Check sheet for the modelled part. Datum: model origin and axes. Units: mm. A direction names the side the tool comes from. Coordinates: 2 decimals unless noted, no trailing zeros. Loops run counter-clockwise (first coordinate to the right, second up) from the corner with the lowest first, then second, coordinate; pieces in that order, holes last. Notation, with made-up numbers: M 30,74 L 48,74 A17 cw 48,100 Z; hole C -3,-3.5 d1. An arc over 180 degrees is marked long. Use CSV: the item, a comma, the result in double quotes. Start each with the question number.
(1) Scan lines: line 1 (X direction, y = 2, z = 6); line 2 (Z direction, x = 3, y = -4); line 3 (Y direction, x = 0, z = 12). Record each from-to range of solid material in increasing order.
(2) Section check A-A on z = 7.5. Record the cut outline in (x, y), and give its area (3 significant figures).
(3) Go/stop test with flat-tipped pins: pin 1 Ø10.5 at (x, y) = (-2, -0.5) entering from -Z; pin 2 Ø5 at (y, z) = (3, 11.5) entering from +X; pin 3 Ø2 at (y, z) = (-2, 16.5) entering from +X; pin 4 Ø4 at (y, z) = (3.5, 4) entering from -X. Record where each tip stops, or that it passes through.
(4) Set-up check for faces 4 (the flat face through (0, 0, 16)), 5 (the cylindrical face through (-0.272, 6.494, 4.93)), 6 (the cylindrical face through (2.5, -1.6, 20)): record each of +Z, -Z, +X, -X, +Y, -Y from which the full face is reachable in a straight line by a thin tool's end or side.
(5) Section check D-D on z = 13. Record the cut outline in (x, y).
(6) Section check B-B on y = 0. Record the cut outline in (x, z).
(7) Section check C-C on x = 0. Record the cut outline in (y, z).
(8) Draft check along X on faces 1 (the flat face through (-2, 7.4, 7)), 2 (the cylindrical face through (-7.493, 0.33, 10.944)), 3 (the flat face through (2, -3, 19)). Enter one of: pulls with the +X half, pulls with the -X half, needs draft (parallel to the pull), parting line crosses it, or undercut.
from build123d import *

# Parameters (mm, degrees)
SKETCH_1_R           = 7.5
EXTRUDE_1_DEPTH      = 5
SKETCH_2_R           = 9
EXTRUDE_2_DEPTH      = 2
SKETCH_3_R           = 7.5
EXTRUDE_3_DEPTH      = 9
CUT_EXTRUDE_1_DEPTH  = 10
SKETCH_4_R           = 1.2
EXTRUDE_4_DEPTH      = 5
EXTRUDE_4_DEPTH_BACK = 14
CUT_EXTRUDE_2_DEPTH  = 2
FILLET_1_R           = 1
FILLET_2_R           = 1


with BuildPart() as part:
    # Sketch 1 → Extrude 1 (new body)
    with BuildSketch(Plane.XY):
        Circle(SKETCH_1_R)
    extrude(amount=EXTRUDE_1_DEPTH)

    # Sketch 2 → Extrude 2 (add)
    with BuildSketch(Plane.XY.offset(5)):
        Circle(SKETCH_2_R)
    extrude(amount=EXTRUDE_2_DEPTH)

    # Sketch 3 → Extrude 3 (add)
    with BuildSketch(Plane.XY.offset(7)):
        Circle(SKETCH_3_R)
    extrude(amount=EXTRUDE_3_DEPTH)

    # Sketch 5 → Cut-Extrude 1 (cut)
    with BuildSketch(Plane(origin=(0, 0, 0), x_dir=(-1, 0, 0), z_dir=(0, 0, -1))):
        with BuildLine():
            ThreePointArc((0.997037031, -6.423076923), (0, 6.5), (-0.997037031, -6.423076923))
            ThreePointArc((-0.997037031, -6.423076923), (0, -5.5), (0.997037031, -6.423076923))
        make_face()
    extrude(amount=-CUT_EXTRUDE_1_DEPTH, mode=Mode.SUBTRACT)

    # Sketch 4 → Extrude 4 (add, two sides)
    with BuildSketch(Plane.XY.offset(16)) as extrude_4_sk:
        with Locations((-2.5, 2.5)):
            Circle(SKETCH_4_R)
        with Locations((-2.5, -2.5)):
            Circle(SKETCH_4_R)
        with Locations((2.5, -2.5)):
            Circle(SKETCH_4_R)
        with Locations((2.5, 2.5)):
            Circle(SKETCH_4_R)
    extrude(amount=EXTRUDE_4_DEPTH)
    extrude(extrude_4_sk.sketch, amount=-EXTRUDE_4_DEPTH_BACK)

    # Sketch 6 → Cut-Extrude 2 (cut)
    with BuildSketch(Plane.XY.offset(21)):
        with BuildLine():
            Line((-4.065638272, 2.5), (-3.4, 2.5))
            ThreePointArc((-3.4, 2.5), (-2.5, 3.4), (-1.6, 2.5))
            Line((-1.6, 2.5), (-1.02269763, 2.5))
            Line((-1.02269763, 2.5), (-1.813265542, 1.11023828))
            Line((-1.813265542, 1.11023828), (-3.304903111, 1.11023828))
            Line((-3.304903111, 1.11023828), (-4.065638272, 2.5))
        make_face()
        with BuildLine():
            Line((1.6, 2.5), (1.02269763, 2.5))
            Line((1.02269763, 2.5), (1.813265542, 1.11023828))
            Line((1.813265542, 1.11023828), (3.304903111, 1.11023828))
            Line((3.304903111, 1.11023828), (4.065638272, 2.5))
            Line((4.065638272, 2.5), (3.4, 2.5))
            ThreePointArc((3.4, 2.5), (2.5, 3.4), (1.6, 2.5))
        make_face()
        with BuildLine():
            Line((4.065638272, -2.5), (3.4, -2.5))
            ThreePointArc((3.4, -2.5), (2.5, -1.6), (1.6, -2.5))
            Line((1.6, -2.5), (1.02269763, -2.5))
            Line((1.02269763, -2.5), (1.813265542, -3.88976172))
            Line((1.813265542, -3.88976172), (3.304903111, -3.88976172))
            Line((3.304903111, -3.88976172), (4.065638272, -2.5))
        make_face()
        with BuildLine():
            Line((-1.02269763, -2.5), (-1.813265542, -3.88976172))
            Line((-1.813265542, -3.88976172), (-3.304903111, -3.88976172))
            Line((-3.304903111, -3.88976172), (-4.065638272, -2.5))
            Line((-4.065638272, -2.5), (-3.4, -2.5))
            ThreePointArc((-3.4, -2.5), (-2.5, -1.6), (-1.6, -2.5))
            Line((-1.6, -2.5), (-1.02269763, -2.5))
        make_face()
    extrude(amount=-CUT_EXTRUDE_2_DEPTH, mode=Mode.SUBTRACT)

    # Fillet 1
    fillet_1_edges = [part.edges().sort_by_distance(p)[0] for p in [
        (-3.7, 2.5, 2),
        (-3.7, -2.5, 2),
        (1.3, -2.5, 2),
        (1.3, 2.5, 2),
    ]]
    fillet(fillet_1_edges, radius=FILLET_1_R)

    # Fillet 2
    fillet_2_edges = [part.edges().sort_by_distance(p)[0] for p in [
        (-7.5, 0, 16),
    ]]
    fillet(fillet_2_edges, radius=FILLET_2_R)


solid = part.part
Outcome:
1,line 1,"x = -8.77 to -6.18, -3.59 to -1.41, 1.41 to 3.59, 6.18 to 8.77"
1,line 2,"z = 10 to 16"
1,line 3,"y = -7.5 to 7.5"
2,outline,"C 0,0 d15; C -2.5,-2.5 d2.4; C -2.5,2.5 d2.4; C 2.5,-2.5 d2.4; C 2.5,2.5 d2.4; hole M -1,-6.42 A1 cw 1,-6.42 A6.5 ccw long Z"
2,area,"63.6 mm²"
3,pin 1,"stops at z = 0"
3,pin 2,"stops at x = 7.48"
3,pin 3,"stops at x = 7.14"
3,pin 4,"stops at x = -8.82"
4,face 4,"+Z"
4,face 5,"-Z"
4,face 6,"+Z, -Y"
5,outline,"C 0,0 d15"
6,outline,"M -9,5 L -7.5,5 L -7.5,0 L -6.5,0 L -6.5,10 L 6.5,10 L 6.5,0 L 7.5,0 L 7.5,5 L 9,5 L 9,7 L 7.5,7 L 7.5,15 A1 ccw 6.5,16 L -6.5,16 A1 ccw -7.5,15 L -7.5,7 L -9,7 Z"
7,outline,"M -9,5 L -7.5,5 L -7.5,0 L -5.5,0 L -5.5,10 L 6.5,10 L 6.5,0 L 7.5,0 L 7.5,5 L 9,5 L 9,7 L 7.5,7 L 7.5,15 A1 ccw 6.5,16 L -6.5,16 A1 ccw -7.5,15 L -7.5,7 L -9,7 Z"
8,face 1,"needs draft"
8,face 2,"parting line crosses it"
8,face 3,"undercut"
